Input: part model. Units: mm. Frame: model coordinates. Give positions to 0.01 mm unless a question says otherwise; leave off trailing zeros. Write each loop counter-clockwise with the first axis right and the second up, starting at its lowest first coordinate (ties: lowest second). Pieces come first, ordered by that corner, then holes. Notation, with made-up numbers: (-35.5, 41.5) - (-13.5, 41.5) arc R18 cw to (-13.5, 52.5) - close; hole circle Ø2 at (23.25, 11.25). An arc over 180 degrees is marked (long way). Answer as CSV lines item,"result".
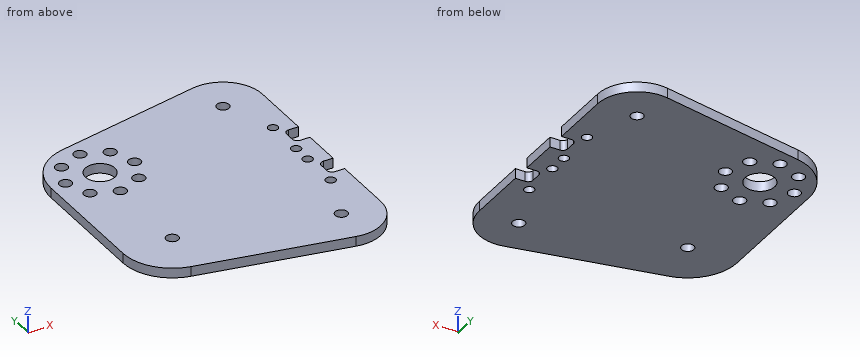
```python
from build123d import *

# Parameters (mm, degrees)
SKETCH_1_R      = 3
SKETCH_1_R_2    = 1.25
SKETCH_1_R_3    = 1
EXTRUDE_2_DEPTH = 2


with BuildPart() as part:
    # 草圖1 → 填料-伸長2 (new body)
    with BuildSketch(Plane.XY):
        with BuildLine():
            Line((-28.541905067, -16.1179941), (-28.541905067, -41.1179941))
            ThreePointArc((-28.541905067, -41.1179941), (-26.279428563, -47.452876116), (-20.515759037, -50.921253788))
            Line((-20.515759037, -50.921253788), (9.479011757, -56.960601851))
            ThreePointArc((9.479011757, -56.960601851), (16.126000545, -55.308012897), (19.058094933, -49.1179941))
            Line((19.058094933, -49.1179941), (19.058094933, -36.6179941))
            Line((19.058094933, -36.6179941), (17.058094933, -36.6179941))
            ThreePointArc((17.058094933, -36.6179941), (16.350988152, -36.325100881), (16.058094933, -35.6179941))
            Line((16.058094933, -35.6179941), (16.058094933, -33.6179941))
            ThreePointArc((16.058094933, -33.6179941), (16.350988152, -32.910887319), (17.058094933, -32.6179941))
            Line((17.058094933, -32.6179941), (19.058094933, -32.6179941))
            Line((19.058094933, -32.6179941), (19.058094933, -24.6179941))
            Line((19.058094933, -24.6179941), (17.058094933, -24.6179941))
            ThreePointArc((17.058094933, -24.6179941), (16.350988152, -24.325100881), (16.058094933, -23.6179941))
            Line((16.058094933, -23.6179941), (16.058094933, -21.6179941))
            ThreePointArc((16.058094933, -21.6179941), (16.350988152, -20.910887319), (17.058094933, -20.6179941))
            Line((17.058094933, -20.6179941), (19.058094933, -20.6179941))
            Line((19.058094933, -20.6179941), (19.058094933, -8.1179941))
            ThreePointArc((19.058094933, -8.1179941), (16.126000545, -1.927975304), (9.479011757, -0.27538635))
            Line((9.479011757, -0.27538635), (-20.515759037, -6.314734412))
            ThreePointArc((-20.515759037, -6.314734412), (-26.279428563, -9.783112085), (-28.541905067, -16.1179941))
        make_face()
        with Locations((-18.541905067, -16.1179941)):
            Circle(SKETCH_1_R, mode=Mode.SUBTRACT)
        with Locations((-18.541905067, -9.1179941)):
            Circle(SKETCH_1_R_2, mode=Mode.SUBTRACT)
        with Locations((-13.592157599, -11.168246632)):
            Circle(SKETCH_1_R_2, mode=Mode.SUBTRACT)
        with Locations((-11.541905067, -16.1179941)):
            Circle(SKETCH_1_R_2, mode=Mode.SUBTRACT)
        with Locations((-13.592157599, -21.067741569)):
            Circle(SKETCH_1_R_2, mode=Mode.SUBTRACT)
        with Locations((-18.541905067, -23.1179941)):
            Circle(SKETCH_1_R_2, mode=Mode.SUBTRACT)
        with Locations((-23.491652536, -21.067741569)):
            Circle(SKETCH_1_R_2, mode=Mode.SUBTRACT)
        with Locations((-25.541905067, -16.1179941)):
            Circle(SKETCH_1_R_2, mode=Mode.SUBTRACT)
        with Locations((-23.491652536, -11.168246632)):
            Circle(SKETCH_1_R_2, mode=Mode.SUBTRACT)
        with Locations((-18.541905067, -41.1179941)):
            Circle(SKETCH_1_R_2, mode=Mode.SUBTRACT)
        with Locations((11.058094933, -8.1179941)):
            Circle(SKETCH_1_R_2, mode=Mode.SUBTRACT)
        with Locations((11.058094933, -49.1179941)):
            Circle(SKETCH_1_R_2, mode=Mode.SUBTRACT)
        with Locations((15.058094933, -26.6179941)):
            Circle(SKETCH_1_R_3, mode=Mode.SUBTRACT)
        with Locations((15.058094933, -18.6179941)):
            Circle(SKETCH_1_R_3, mode=Mode.SUBTRACT)
        with Locations((15.058094933, -38.6179941)):
            Circle(SKETCH_1_R_3, mode=Mode.SUBTRACT)
        with Locations((15.058094933, -30.6179941)):
            Circle(SKETCH_1_R_3, mode=Mode.SUBTRACT)
    extrude(amount=EXTRUDE_2_DEPTH)


solid = part.part
```
Item 1: Cut plane D-D on x = 8. Return the cut outline in (y, z), plus the area to 3 significant figures.
The answers:
outline,"(-56.66, 0) - (-0.57, 0) - (-0.57, 2) - (-56.66, 2) - close"
area,"112 mm²"
Item 2: Contact query for flat-ended pins moving along their axis: pin 1 (1.8 mm diameter, centred on x = 15.06, y = -38.62, fed in from -Z); pin 2 (0.6 mm diameter, centred on x = 18, z = 1, fed in from -Y); pin 3 (0.6 mm diameter, centred on y = -34.5, z = 0.5, fed in from +X). Output: stop coordinate, or through.
The answers:
pin 1,"through"
pin 2,"y = -53.58"
pin 3,"x = 16.06"
Item 3: Cut plane C-C on y = -4.5. Return the cut outline in (x, z), plus the area to 3 significant figures.
The answers:
outline,"(-11.5, 0) - (18.19, 0) - (18.19, 2) - (-11.5, 2) - close"
area,"59.4 mm²"
Item 4: Ray query, line 1 (X direction, y = -16, z = 1.4); line 2 (X direction, y = -18, z = 0.45); line 3 (X direction, y = -20, z = 0.75). Return the intervals inside material, ascending. Write a range as from..to.
The answers:
line 1,"-28.54..-26.79, -24.3..-21.54, -15.54..-12.79, -10.3..19.06"
line 2,"-28.54..-20.88, -16.21..14.27, 15.84..19.06"
line 3,"-28.54..-24.14, -22.84..-14.24, -12.94..19.06"
Item 5: Cut plane A-A on x = -16.5. Return the cut outline in (y, z), plus the area to 3 significant figures.
The answers:
outline,"(-51.73, 0) - (-18.32, 0) - (-18.32, 2) - (-51.73, 2) - close; (-13.92, 0) - (-5.51, 0) - (-5.51, 2) - (-13.92, 2) - close"
area,"83.7 mm²"
Item 6: Cut plane B-B on z = 0.75. Count the separate pieces of the cut face and the enclosed holes in it, plus the area to 3 significant figures.
The answers:
separate pieces,"1"
enclosed holes,"16"
area,"2,240 mm²"
